Design review of the part built by this model. Coordinates are the model's own, in mm. Give positions to 0.01 mm unless a question says otherwise; leave off trailing zeros. Loops run counter-clockwise (first coordinate to the right, second up) from the corner with the lowest first, then second, coordinate; pieces in that order, holes last. Notation, with made-up numbers: (23, 89) - (56, 89) arc R18 ccw to (56, 100) - close; hole circle Ø3 at (64.25, -15). An arc over 180 degrees is marked (long way). One line per item, written item: value. Start each with the question number.
```python
from build123d import *

# Parameters (mm, degrees)
PLATE_EXTRUDE_1_DEPTH             = 3
M6_TAPPED_HOLE2_AT_2_COUNT        = 2
M6_TAPPED_HOLE2_AT_2_PITCH        = 300
M6_TAPPED_HOLE2_AT_3_COUNT        = 2
M6_TAPPED_HOLE2_AT_3_PITCH        = 180.277563773
M6_TAPPED_HOLE2_AT_4_COUNT        = 2
M6_TAPPED_HOLE2_AT_4_PITCH        = 200.51462203
M6_TAPPED_HOLE2_AT_5_COUNT        = 2
M6_TAPPED_HOLE2_AT_5_PITCH        = 360.55459645
TAP_DRILL_FOR_M6_TAP1_D           = 5
TAP_DRILL_FOR_M6_TAP1_DEPTH       = 10
TAP_DRILL_FOR_M6_TAP1_CSINK_D     = 5.05
TAP_DRILL_FOR_M6_TAP1_CSINK_ANGLE = 90
TAP_DRILL_FOR_M6_TAP1_TIP         = 1.502151548


with BuildPart() as part:
    # Plate Template → Plate Extrude 1 (new body)
    with BuildSketch(Plane(origin=(0, 0, 0), x_dir=(1, 0, 0), z_dir=(0, 1, 0))):
        with BuildLine():
            Line((-79.570676183, 225.004191897), (79.570676183, 225.004191897))
            ThreePointArc((79.570676183, 225.004191897), (79.965179487, 224.92308642), (80.295690033, 224.692926184))
            Line((80.295690033, 224.692926184), (174.72501385, 125.289471239))
            ThreePointArc((174.72501385, 125.289471239), (174.928712509, 124.971537539), (175, 124.600736953))
            Line((175, 124.600736953), (175, -124))
            ThreePointArc((175, -124), (174.707106781, -124.707106781), (174, -125))
            Line((174, -125), (-174, -125))
            ThreePointArc((-174, -125), (-174.707106781, -124.707106781), (-175, -124))
            Line((-175, -124), (-175, 124.600736953))
            ThreePointArc((-175, 124.600736953), (-174.928712509, 124.971537539), (-174.72501385, 125.289471239))
            Line((-174.72501385, 125.289471239), (-80.295690033, 224.692926184))
            ThreePointArc((-80.295690033, 224.692926184), (-79.965179487, 224.92308642), (-79.570676183, 225.004191897))
        make_face()
    extrude(amount=PLATE_EXTRUDE_1_DEPTH)

    # Sketch3 → M6 Tapped Hole2 (revolve, cut)
    with BuildSketch(Plane(origin=(-150, 3, 100), x_dir=(0, 0, 1), z_dir=(1, 0, 0))):
        Polygon((0, 0), (0, 3), (2.5, 3), (2.5, 0.525), (3.025, 0), align=None)
    m6_tapped_hole2 = revolve(axis=Axis((-150, 9.35, 100), (0, -1, 0)), mode=Mode.SUBTRACT)

    # M6 Tapped Hole2 at 2: M6 Tapped Hole2 ×2
    with Locations(*[(i * M6_TAPPED_HOLE2_AT_2_PITCH, 0, 0) for i in range(1, M6_TAPPED_HOLE2_AT_2_COUNT)]):
        add(m6_tapped_hole2, mode=Mode.SUBTRACT)

    # M6 Tapped Hole2 at 3: M6 Tapped Hole2 ×2
    with Locations(*[Vector(0.8320502943378437, 0, -0.554700196225229) * (i * M6_TAPPED_HOLE2_AT_3_PITCH) for i in range(1, M6_TAPPED_HOLE2_AT_3_COUNT)]):
        add(m6_tapped_hole2, mode=Mode.SUBTRACT)

    # M6 Tapped Hole2 at 4: M6 Tapped Hole2 ×2
    with Locations(*[Vector(0.0017163887650713508, 0, -0.9999985270037187) * (i * M6_TAPPED_HOLE2_AT_4_PITCH) for i in range(1, M6_TAPPED_HOLE2_AT_4_COUNT)]):
        add(m6_tapped_hole2, mode=Mode.SUBTRACT)

    # M6 Tapped Hole2 at 5: M6 Tapped Hole2 ×2
    with Locations(*[Vector(0.8330011499156382, 0, -0.5532712573767269) * (i * M6_TAPPED_HOLE2_AT_5_PITCH) for i in range(1, M6_TAPPED_HOLE2_AT_5_COUNT)]):
        add(m6_tapped_hole2, mode=Mode.SUBTRACT)

    # Tap Drill for M6 Tap1
    with Locations(Plane(origin=(0, 0, 0), x_dir=(-1, 0, 0), z_dir=(0, -1, 0))):
        with Locations((-46.5, 191.004191906), (32.5, 191.004191906), (32.5, 99.004191897), (-46.5, 99.004191897)):
            CounterSinkHole(TAP_DRILL_FOR_M6_TAP1_D / 2, TAP_DRILL_FOR_M6_TAP1_CSINK_D / 2, depth=TAP_DRILL_FOR_M6_TAP1_DEPTH, counter_sink_angle=TAP_DRILL_FOR_M6_TAP1_CSINK_ANGLE)
            with Locations((0, 0, -(TAP_DRILL_FOR_M6_TAP1_DEPTH + TAP_DRILL_FOR_M6_TAP1_TIP / 2))):  # 118° drill point
                Cone(0, TAP_DRILL_FOR_M6_TAP1_D / 2, TAP_DRILL_FOR_M6_TAP1_TIP, mode=Mode.SUBTRACT)


solid = part.part
```
(1) Take a section at B-B on z = -152. State the section outline as (x, y) points.
(2) Take a section at A-A on x = 98.5. State the section outline as (y, z) points.
(3) To check wall thickness, follow L1, parallel to X at y = 1.5, z = 100; L2, parallel to Z at x = -150, y = 0.7; L3, parallel to Z at x = 46.5, y = 1.9. State the ranges of each line that lie inside material, in increasing order. Write a range as from..to.
(4) For pin 1 Ø4.5 at (x, z) = (46.5, -99) entering from +Y, flat-tipped, find the tip position at first contact; note if it passes through.
Here are the results:
1. outline: (-149.35, 0) - (149.35, 0) - (149.35, 3) - (-149.35, 3) - close
2. outline: (0, -205.53) - (3, -205.53) - (3, 125) - (0, 125) - close
3. L1: -175..-152.5, -147.5..147.5, 152.5..175
3. L2: -151.32..-102.99, -98.04..97.5, 102.5..125
3. L3: -225..-193.5, -188.5..-101.5, -96.5..125
4. pin 1: through
